Source: CAD feature listing. Evaluate the final solid. Frame: model axes, mm. A direction names the side the tool comes from. Give positions to 0.01 mm unless a question says otherwise; leave off trailing zeros. Loops run counter-clockwise (first coordinate to the right, second up) from the corner with the lowest first, then second, coordinate; pieces in that order, holes last. Notation, with made-up numbers: (-11.75, 40) - (34.25, 40) arc R23 cw to (34.25, 52) - close; hole circle Ø7 at (83.25, -29). An arc over 180 degrees is marked (long way). Put each result on its own line as item: value.
```python
from build123d import *

# Parameters (mm, degrees)
F1_DEPTH = 10
F3_D     = 3.3
F4_D     = 3.3


with BuildPart() as f1:
    # F0 (on Right) → F1 (new body)
    with BuildSketch(Plane.YZ):
        with BuildLine():
            ThreePointArc((-22.8023384852, 19.4527051061), (-15.9795824438, 32.7527051061), (-9.1568264025, 19.4527051061))
            Line((-9.1568264025, 19.4527051061), (-5.1476741432, 19.4527051061))
            ThreePointArc((-5.1476741432, 19.4527051061), (-15.6627106592, 35.6093140728), (-26.1777471751, 19.4527051061))
            Line((-26.1777471751, 19.4527051061), (-22.8023384852, 19.4527051061))
        make_face()
        Polygon((-5.1476741432, 19.4527051061), (-9.1568264025, 19.4527051061), (-9.1568264025, 15.9527051061), (2.8431735975, 15.9527051061), (2.8431735975, 19.4527051061), align=None)
        Polygon((-22.8023384852, 15.9527051061), (-22.8023384852, 19.4527051061), (-26.1777471751, 19.4527051061), (-34.8023384852, 19.4527051061), (-34.8025824438, 15.9527051061), align=None)
    extrude(amount=F1_DEPTH)

    # F3 (through all)
    with Locations(Plane(origin=(0, 0, 0), x_dir=(1, 0, 0), z_dir=(0, 0, -1))):
        with Locations((5.1220096648, 32)):
            Hole(F3_D / 2)

    # F4 (through all)
    with Locations(Plane(origin=(0, 0, 0), x_dir=(1, 0, 0), z_dir=(0, 0, -1))):
        with Locations((5.00610983, 0)):
            Hole(F4_D / 2)


solid = f1.part
```
1) Material intervals for line 1 along Y through (x, z) = (5, 24.5); line 2 along Y through (x, z) = (3.25, 18.5); line 3 along X through (y, z) = (-32, 17.4), sorted ascending. Write a range as [from, to].
Check result:
line 1: [-27.16, -24.38], [-7.58, -4.17]
line 2: [-34.8, -22.8], [-9.16, 2.84]
line 3: [0, 3.47], [6.77, 10]
2) Pin query (flat end, axial travel): P1, Ø3, axis at x = 1.5, z = 32, coming from the -Y side; P2, Ø1, axis at x = 6.5, y = -31, coming from the +Z side; P3, Ø4, axis at x = 6, z = 30, coming from the -Y side. Return the tip coordinate at first contact, or that it passes through.
Check result:
P1: y = -25.22
P2: z = 19.45
P3: y = -26.48
3) Section query C-C, the plane z = 20.5. Output: boundary loops of the cut face in (x, y).
Check result:
outline: (0, -26.58) - (10, -26.58) - (10, -23.44) - (0, -23.44) - close; (0, -8.52) - (10, -8.52) - (10, -4.74) - (0, -4.74) - close
4) Access query for faces 5 (the flat face through (0, -7.7, 22.2)), 6 (the flat face through (5, -2, 19.453)), 7 (the flat face through (5, -29, 15.953)), 8 (the flat face through (5, -22.802, 18)), 9 (the flat face through (5, -29, 19.453)). Directions: +Z, -Z, +X, -X, +Y, -Y. A direction counts if a zero-diameter tool reaches every point of the face in a straight line with its end or side. Return the directions, or none.
Check result:
face 5: +Z, -Z, -X, +Y, -Y
face 6: +X, -X, +Y
face 7: -Z, +X, -X, +Y, -Y
face 8: -Z, +X, -X
face 9: +X, -X, -Y
5) Section query D-D, the plane x = 8.5. Output: boundary loops of the cut face in (y, z), plus the area to 3 significant figures.
Check result:
outline: (-34.8, 15.95) - (-22.8, 15.95) - (-22.8, 19.45) arc R8.4 cw (long way) to (-9.16, 19.45) - (-9.16, 15.95) - (2.84, 15.95) - (2.84, 19.45) - (-5.15, 19.45) arc R11.5 ccw (long way) to (-26.18, 19.45) - (-34.8, 19.45) - close
area: 208 mm²
6) Mould query, pull axis X, two halves, no side actions, for faces 1 (the cylindrical face through (4.93, -16.24, 32.75)), 2 (the flat face through (10, -7.7, 22.2)), 3 (the cylindrical face through (3.432, -0.496, 17.727)), 4 (the cylindrical face through (5.337, -33.636, 17.727)). Classes: pulls with the +X half, pulls with the -X half, needs draft (parallel to the pull), parting line crosses it, or undercut.
Check result:
face 1: needs draft
face 2: pulls with the +X half
face 3: undercut
face 4: undercut
7) Section query A-A, the plane y = -32. Output: boundary loops of the cut face in (x, z), plus the area to 4 significant figures.
Check result:
outline: (0, 15.95) - (3.47, 15.95) - (3.47, 19.45) - (0, 19.45) - close; (6.77, 15.95) - (10, 15.95) - (10, 19.45) - (6.77, 19.45) - close
area: 23.45 mm²
8) Section query B-B, the plane x = 4.75. Output: boundary loops of the cut face in (y, z), plus the area to 3 significant figures.
Check result:
outline: (-34.8, 15.95) - (-33.61, 15.95) - (-33.61, 19.45) - (-34.8, 19.45) - close; (-30.39, 15.95) - (-22.8, 15.95) - (-22.8, 19.45) arc R8.4 cw (long way) to (-9.16, 19.45) - (-9.16, 15.95) - (-1.63, 15.95) - (-1.63, 19.45) - (-5.15, 19.45) arc R11.5 ccw (long way) to (-26.18, 19.45) - (-30.39, 19.45) - close; (1.63, 15.95) - (2.84, 15.95) - (2.84, 19.45) - (1.63, 19.45) - close
area: 185 mm²
